Check sheet for the modelled part. Datum: model origin and axes. Units: mm. Coordinates: 2 decimals unless noted, no trailing zeros. Order: outer loops, then holes, each group sorted by start corner. A loop starts at its lowest first (then second) coordinate and runs counter-clockwise, first axis right, second up.
1. Cross-section at A-A (z = 226.5). Enter the section's corners in (x, y).
2. Cross-section at B-B (x = 86). Enter the section's corners in (y, z), then the cut area to 3 significant figures.
3. Cross-section at C-C (y = 0.5). Count the separate pieces of the cut face and the enclosed holes in it, then the cut area to 3 significant figures.
4. Thickness scan on line 1 (Z direction, x = 25, y = 0.6); line 2 (X direction, y = 1.9, z = 234); line 3 (Z direction, x = -112, y = 1.55). Record the ranges inside material, lowest first.
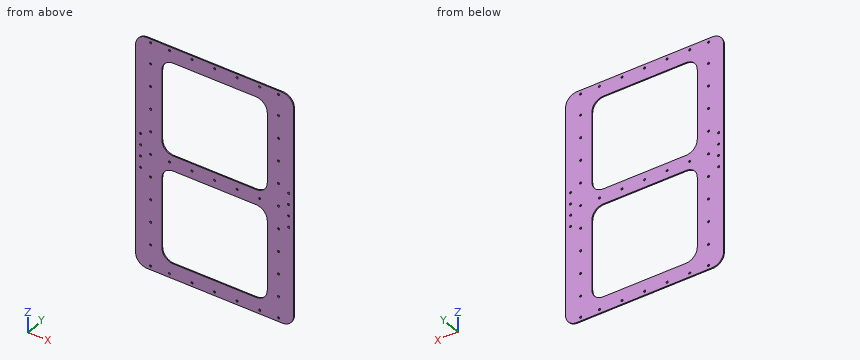
```python
from build123d import *

# Parameters (mm, degrees)
SKETCH1_W               = 420
SKETCH1_H               = 612
BOSS_EXTRUDE1_DEPTH     = 3
SKETCH_1_R              = 2.75
CUT_EXTRUDE_1_DEPTH     = 372.140135259
CUT_EXTRUDE1_DEPTH      = 372.140135259
CUT_EXTRUDE1_DEPTH_BACK = 372.140135259
SKETCH2_W               = 280
SKETCH2_H               = 246
FILLET1_R               = 30
FILLET2_R               = 30


with BuildPart() as part:
    # Sketch1 → Boss-Extrude1 (new body)
    with BuildSketch(Plane(origin=(0, 0, 0), x_dir=(1, 0, 0), z_dir=(0, 1, 0))):
        Rectangle(SKETCH1_W, SKETCH1_H)
    extrude(amount=BOSS_EXTRUDE1_DEPTH)

    # 草图1 → 切除-拉伸1 (cut, through all)
    with BuildSketch(Plane(origin=(0, 3, 0), x_dir=(1, 0, 0), z_dir=(0, 1, 0))):
        with Locations(Location((-170, 240, 0), (0, 0, 270))):
            Circle(SKETCH_1_R)
        with Locations(Location((-170, 180, 0), (0, 0, 270))):
            Circle(SKETCH_1_R)
        with Locations(Location((-196.85, -15, 0), (0, 0, 270))):
            Circle(SKETCH_1_R)
        with Locations(Location((-196.85, -45, 0), (0, 0, 270))):
            Circle(SKETCH_1_R)
        with Locations(Location((-196.85, 45, 0), (0, 0, 90))):
            Circle(SKETCH_1_R)
        with Locations(Location((-196.85, 15, 0), (0, 0, 90))):
            Circle(SKETCH_1_R)
        with Locations(Location((196.85, 15, 0), (0, 0, 270))):
            Circle(SKETCH_1_R)
        with Locations(Location((196.85, 45, 0), (0, 0, 270))):
            Circle(SKETCH_1_R)
        with Locations(Location((196.85, -45, 0), (0, 0, 90))):
            Circle(SKETCH_1_R)
        with Locations(Location((196.85, -15, 0), (0, 0, 90))):
            Circle(SKETCH_1_R)
        with Locations(Location((0, 0, 0), (0, 0, 270))):
            Circle(SKETCH_1_R)
        with Locations(Location((-60, 0, 0), (0, 0, 270))):
            Circle(SKETCH_1_R)
        with Locations(Location((-120, 0, 0), (0, 0, 270))):
            Circle(SKETCH_1_R)
        with Locations(Location((60, 0, 0), (0, 0, 90))):
            Circle(SKETCH_1_R)
        with Locations(Location((120, 0, 0), (0, 0, 90))):
            Circle(SKETCH_1_R)
        with Locations(Location((0, 296, 0), (0, 0, 270))):
            Circle(SKETCH_1_R)
        with Locations(Location((-60, 296, 0), (0, 0, 270))):
            Circle(SKETCH_1_R)
        with Locations(Location((-120, 296, 0), (0, 0, 270))):
            Circle(SKETCH_1_R)
        with Locations(Location((-170, 296, 0), (0, 0, 270))):
            Circle(SKETCH_1_R)
        with Locations(Location((170, 296, 0), (0, 0, 90))):
            Circle(SKETCH_1_R)
        with Locations(Location((-170, 120, 0), (0, 0, 270))):
            Circle(SKETCH_1_R)
        with Locations(Location((-170, 60, 0), (0, 0, 270))):
            Circle(SKETCH_1_R)
        with Locations(Location((-170, 0, 0), (0, 0, 270))):
            Circle(SKETCH_1_R)
        with Locations(Location((-170, -60, 0), (0, 0, 270))):
            Circle(SKETCH_1_R)
        with Locations(Location((-170, -120, 0), (0, 0, 270))):
            Circle(SKETCH_1_R)
        with Locations(Location((-170, -180, 0), (0, 0, 270))):
            Circle(SKETCH_1_R)
        with Locations(Location((-170, -240, 0), (0, 0, 270))):
            Circle(SKETCH_1_R)
        with Locations(Location((170, -240, 0), (0, 0, 90))):
            Circle(SKETCH_1_R)
        with Locations(Location((170, -180, 0), (0, 0, 90))):
            Circle(SKETCH_1_R)
        with Locations(Location((170, -120, 0), (0, 0, 90))):
            Circle(SKETCH_1_R)
        with Locations(Location((170, -60, 0), (0, 0, 90))):
            Circle(SKETCH_1_R)
        with Locations(Location((170, 0, 0), (0, 0, 90))):
            Circle(SKETCH_1_R)
        with Locations(Location((170, 60, 0), (0, 0, 90))):
            Circle(SKETCH_1_R)
        with Locations(Location((170, 120, 0), (0, 0, 90))):
            Circle(SKETCH_1_R)
        with Locations(Location((170, 180, 0), (0, 0, 90))):
            Circle(SKETCH_1_R)
        with Locations(Location((170, 240, 0), (0, 0, 90))):
            Circle(SKETCH_1_R)
        with Locations(Location((60, 296, 0), (0, 0, 90))):
            Circle(SKETCH_1_R)
        with Locations(Location((120, 296, 0), (0, 0, 90))):
            Circle(SKETCH_1_R)
        with Locations(Location((120, -296, 0), (0, 0, 270))):
            Circle(SKETCH_1_R)
        with Locations(Location((60, -296, 0), (0, 0, 270))):
            Circle(SKETCH_1_R)
        with Locations(Location((170, -296, 0), (0, 0, 270))):
            Circle(SKETCH_1_R)
        with Locations(Location((-170, -296, 0), (0, 0, 90))):
            Circle(SKETCH_1_R)
        with Locations(Location((-120, -296, 0), (0, 0, 90))):
            Circle(SKETCH_1_R)
        with Locations(Location((-60, -296, 0), (0, 0, 90))):
            Circle(SKETCH_1_R)
        with Locations(Location((0, -296, 0), (0, 0, 90))):
            Circle(SKETCH_1_R)
    extrude(amount=-CUT_EXTRUDE_1_DEPTH, mode=Mode.SUBTRACT)

    # Sketch2 → Cut-Extrude1 (cut, two sides: drawn at the far end of the back side and taken through both)
    with BuildSketch(Plane(origin=(0, 3, 0), x_dir=(1, 0, 0), z_dir=(0, 1, 0)).offset(-CUT_EXTRUDE1_DEPTH_BACK)):
        with Locations((0, 143)):
            Rectangle(SKETCH2_W, SKETCH2_H)
        with Locations((0, -143)):
            Rectangle(SKETCH2_W, SKETCH2_H)
    extrude(amount=CUT_EXTRUDE1_DEPTH + CUT_EXTRUDE1_DEPTH_BACK, mode=Mode.SUBTRACT)

    # Fillet1
    fillet1_edges = [part.edges().sort_by_distance(p)[0] for p in [
        (140, 1.5, -266),
        (140, 1.5, -20),
        (-140, 1.5, -20),
        (-140, 1.5, -266),
        (-140, 1.5, 266),
        (-140, 1.5, 20),
        (140, 1.5, 20),
        (140, 1.5, 266),
    ]]
    fillet(fillet1_edges, radius=FILLET1_R)

    # Fillet2
    fillet2_edges = [part.edges().sort_by_distance(p)[0] for p in [
        (210, 1.5, 306),
        (-210, 1.5, 306),
        (-210, 1.5, -306),
        (210, 1.5, -306),
    ]]
    fillet(fillet2_edges, radius=FILLET2_R)


solid = part.part
```
Data:
1. outline: (-210, 0) - (-140, 0) - (-140, 3) - (-210, 3) - close; (140, 0) - (210, 0) - (210, 3) - (140, 3) - close
2. outline: (0, -306) - (3, -306) - (3, -266) - (0, -266) - close; (0, -20) - (3, -20) - (3, 20) - (0, 20) - close; (0, 266) - (3, 266) - (3, 306) - (0, 306) - close
2. area: 360 mm2
3. separate pieces: 1
3. enclosed holes: 47
3. area: 119,000 mm2
4. line 1: z = -306 to -266, -20 to 20, 266 to 306
4. line 2: x = -210 to -140, 140 to 210
4. line 3: z = -306 to -265.93, -20.07 to 20.07, 265.93 to 306
